Geometry: final body of the model. Coordinates: model frame, mm. Face numbers are marked on the shaded views. A direction names the side the tool comes from. Give positions to 0.01 mm unless a question says otherwise; leave off trailing zeros. Write each loop counter-clockwise with the first axis right and the second up, starting at its lowest first coordinate (ties: lowest second). Pieces come first, ordered by that corner, then holes. Notation, with made-up numbers: (-20, 12) -> (33, 12) arc R26 cw to (33, 36) -> close; hole circle Ø10 at (-8.75, 8.5). An arc over 180 degrees is marked (long way). Answer in a Markdown table with one row per item. Add a question column.
Item 1: Section query A-A on y = 0. Output: boundary loops of the cut face in (x, z).
Item 2: Access query for the marked faces 1 and 2. Directions: +Z, -Z, +X, -X, +Y, -Y. A direction counts if a zero-diameter tool reaches every point of the face in a straight line with its end or side. Return the directions, or none.
Item 3: Section query D-D on z = 1.25. Output: boundary loops of the cut face in (x, y).
Item 4: Material intervals for probe 1 along Y at (x, z) = (0, 2); probe 2 along Z at (x, y) = (-1.5, -18); probe 3 along Y at (x, z) = (0, -3.75), sorted ascending. Write a range as from..to.
Item 5: First-contact query: P1, Ø6.5, axis at x = -24.86, y = 28.08, coming from the -Z side; P2, Ø6, axis at y = 15, z = -7.5, coming from the -X side; P3, Ø11, axis at x = 24.86, y = 28.08, coming from the -Z side; P4, Ø12, axis at y = 13.5, z = -11.5, coming from the -X side. Flat tips, straight axial feed; report the tip coordinate or a pass-through.
Item 6: Section query C-C on z = -3.75. Output: boundary loops of the cut face in (x, y), plus the area to 3 significant figures.
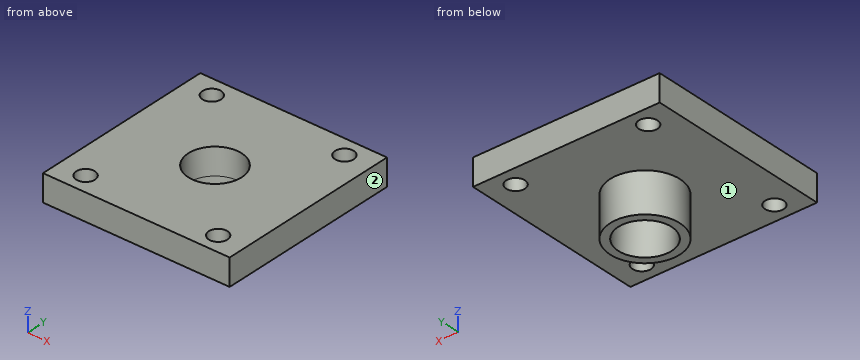
```python
from build123d import *

# Parameters (mm, degrees)
SKETCH1_W           = 70
SKETCH1_H           = 70
BOSS_EXTRUDE1_DEPTH = 10
SKETCH2_R           = 10
CUT_EXTRUDE1_DEPTH  = 10
SKETCH4_R           = 3.5
CUT_EXTRUDE2_DEPTH  = 35
SKETCH5_R           = 13.071961786
SKETCH5_R_2         = 10
BOSS_EXTRUDE3_DEPTH = 15


with BuildPart() as part:
    # Sketch1 → Boss-Extrude1 (new body)
    with BuildSketch(Plane.XY):
        Rectangle(SKETCH1_W, SKETCH1_H)
    extrude(amount=BOSS_EXTRUDE1_DEPTH)

    # Sketch2 → Cut-Extrude1 (cut)
    with BuildSketch(Plane.XY.offset(10)):
        Circle(SKETCH2_R)
    extrude(amount=-CUT_EXTRUDE1_DEPTH, mode=Mode.SUBTRACT)

    # Sketch4 → Cut-Extrude2 (cut)
    with BuildSketch(Plane(origin=(0, 0, 0), x_dir=(-1, 0, 0), z_dir=(0, 0, -1))):
        with Locations((-24.855592085, 28.07934369)):
            Circle(SKETCH4_R)
        with Locations((24.855592085, 28.07934369)):
            Circle(SKETCH4_R)
        with Locations((24.855592085, -28.07934369)):
            Circle(SKETCH4_R)
        with Locations((-24.855592085, -28.07934369)):
            Circle(SKETCH4_R)
    extrude(amount=-CUT_EXTRUDE2_DEPTH, mode=Mode.SUBTRACT)

    # Sketch5 → Boss-Extrude3 (add)
    with BuildSketch(Plane(origin=(0, 0, 0), x_dir=(-1, 0, 0), z_dir=(0, 0, -1))):
        with Locations(Location((0, 0, 0), (0, 0, 180))):
            Circle(SKETCH5_R)
        with Locations(Location((0, 0, 0), (0, 0, 180))):
            Circle(SKETCH5_R_2, mode=Mode.SUBTRACT)
    extrude(amount=BOSS_EXTRUDE3_DEPTH)


solid = part.part
```
Findings below:
| question | item | result |
|---|---|---|
| 1 | outline | (-35, 0) -> (-13.07, 0) -> (-13.07, -15) -> (-10, -15) -> (-10, 10) -> (-35, 10) -> close; (10, -15) -> (13.07, -15) -> (13.07, 0) -> (35, 0) -> (35, 10) -> (10, 10) -> close |
| 2 | face 1 | -Z |
| 2 | face 2 | +Z, -Z, +X, +Y, -Y |
| 3 | outline | (-35, -35) -> (35, -35) -> (35, 35) -> (-35, 35) -> close; hole circle Ø7 at (-24.86, -28.08); hole circle Ø7 at (-24.86, 28.08); hole circle Ø20 at (0, 0); hole circle Ø7 at (24.86, -28.08); hole circle Ø7 at (24.86, 28.08) |
| 4 | probe 1 | y = -35..-10, 10..35 |
| 4 | probe 2 | z = 0..10 |
| 4 | probe 3 | y = -13.07..-10, 10..13.07 |
| 5 | P1 | passes through |
| 5 | P2 | stops at x = -5.18 |
| 5 | P3 | stops at z = 0 |
| 5 | P4 | stops at x = -10.71 |
| 6 | outline | circle Ø26.14 at (0, 0); hole circle Ø20 at (0, 0) |
| 6 | area | 223 mm^2 |
